from build123d import *

# Parameters (mm, degrees)
BOSS_EXTRUDE1_DEPTH      = 54.6167
BOSS_EXTRUDE1_DEPTH_BACK = 45.3833
SKETCH2_W                = 20
SKETCH2_H                = 20
CUT_EXTRUDE1_DEPTH       = 91
SKETCH3_W                = 20
SKETCH3_H                = 20
CUT_EXTRUDE2_DEPTH       = 91
BOSS_EXTRUDE2_START      = -45.3833
SKETCH1_5_W              = 3
SKETCH1_5_H              = 10
SKETCH1_5_W_2            = 10
SKETCH1_5_H_2            = 3
BOSS_EXTRUDE2_DEPTH      = 80
CUT_EXTRUDE3_REACH       = 92
SKETCH5_R                = 5
SKETCH5_R_2              = 3.4
CUT_EXTRUDE4_REACH       = 92
SKETCH4_R                = 5
SKETCH4_R_2              = 3.4


with BuildPart() as part:
    # Sketch1 → Boss-Extrude1 (new body, two sides)
    with BuildSketch(Plane(origin=(0, 0, 0), x_dir=(1, 0, 0), z_dir=(0, 1, 0))) as boss_extrude1_sk:
        with BuildLine():
            ThreePointArc((45, 25), (39.142135624, 39.142135624), (25, 45))
            Line((25, 45), (-25, 45))
            ThreePointArc((-25, 45), (-39.142135624, 39.142135624), (-45, 25))
            Line((-45, 25), (-45, -25))
            ThreePointArc((-45, -25), (-39.142135624, -39.142135624), (-25, -45))
            Line((-25, -45), (25, -45))
            Line((25, -45), (25, -38))
            Line((25, -38), (15, -38))
            Line((15, -38), (5, -38))
            Line((5, -38), (5, -35))
            Line((5, -35), (-25, -35))
            ThreePointArc((-25, -35), (-32.071067812, -32.071067812), (-35, -25))
            Line((-35, -25), (-35, 25))
            ThreePointArc((-35, 25), (-32.071067812, 32.071067812), (-25, 35))
            Line((-25, 35), (25, 35))
            ThreePointArc((25, 35), (32.071067812, 32.071067812), (35, 25))
            Line((35, 25), (35, -5))
            Line((35, -5), (38, -5))
            Line((38, -5), (38, -15))
            Line((38, -15), (38, -25))
            Line((38, -25), (45, -25))
            Line((45, -25), (45, 25))
        make_face()
    extrude(amount=BOSS_EXTRUDE1_DEPTH)
    extrude(boss_extrude1_sk.sketch, amount=-BOSS_EXTRUDE1_DEPTH_BACK)

    # Sketch2 → Cut-Extrude1 (cut, through all)
    with BuildSketch(Plane(origin=(0, 0, -45), x_dir=(-1, 0, 0), z_dir=(0, 0, -1))):
        with Locations((-35, 44.616700276)):
            Rectangle(SKETCH2_W, SKETCH2_H)
    extrude(amount=-CUT_EXTRUDE1_DEPTH, mode=Mode.SUBTRACT)

    # Sketch3 → Cut-Extrude2 (cut, through all)
    with BuildSketch(Plane.ZY.offset(45)):
        with Locations((35, 44.616700276)):
            Rectangle(SKETCH3_W, SKETCH3_H)
    extrude(amount=-CUT_EXTRUDE2_DEPTH, mode=Mode.SUBTRACT)

    # Sketch1<5> → Boss-Extrude2 (add)
    with BuildSketch(Plane(origin=(0, 0, 0), x_dir=(1, 0, 0), z_dir=(0, 1, 0)).offset(BOSS_EXTRUDE2_START)):
        with BuildLine():
            Line((25, -25), (35, -25))
            Line((35, -25), (35, -15))
            Line((35, -15), (25, -15))
            ThreePointArc((25, -15), (17.928932188, -17.928932188), (15, -25))
            Line((15, -25), (15, -35))
            Line((15, -35), (25, -35))
            Line((25, -35), (25, -25))
        make_face()
        with Locations((36.5, -20)):
            Rectangle(SKETCH1_5_W, SKETCH1_5_H)
        with Locations((20, -36.5)):
            Rectangle(SKETCH1_5_W_2, SKETCH1_5_H_2)
    extrude(amount=BOSS_EXTRUDE2_DEPTH)

    # Sketch5 → Cut-Extrude3 (cut, up to next)
    with BuildSketch(Plane(origin=(0, 0, -45), x_dir=(-1, 0, 0), z_dir=(0, 0, -1)), mode=Mode.PRIVATE) as cut_extrude3_sk1:
        with Locations((0, 9.016700277)):
            Circle(SKETCH5_R)
    cut_extrude3_tool1 = extrude(cut_extrude3_sk1.sketch, amount=-CUT_EXTRUDE3_REACH, mode=Mode.PRIVATE) & part.part
    add(cut_extrude3_tool1.solids().sort_by_distance((0, 9.0167, -45))[0], mode=Mode.SUBTRACT)
    # Sketch5 → Cut-Extrude3 (cut, up to next)
    with BuildSketch(Plane(origin=(0, 0, -45), x_dir=(-1, 0, 0), z_dir=(0, 0, -1)), mode=Mode.PRIVATE) as cut_extrude3_sk2:
        with Locations((0, -25.983299723)):
            Circle(SKETCH5_R)
    cut_extrude3_tool2 = extrude(cut_extrude3_sk2.sketch, amount=-CUT_EXTRUDE3_REACH, mode=Mode.PRIVATE) & part.part
    add(cut_extrude3_tool2.solids().sort_by_distance((0, -25.9833, -45))[0], mode=Mode.SUBTRACT)
    # Sketch5 → Cut-Extrude3 (cut, up to next)
    with BuildSketch(Plane(origin=(0, 0, -45), x_dir=(-1, 0, 0), z_dir=(0, 0, -1)), mode=Mode.PRIVATE) as cut_extrude3_sk3:
        with Locations((16, -25.983299723)):
            Circle(SKETCH5_R_2)
    cut_extrude3_tool3 = extrude(cut_extrude3_sk3.sketch, amount=-CUT_EXTRUDE3_REACH, mode=Mode.PRIVATE) & part.part
    add(cut_extrude3_tool3.solids().sort_by_distance((-16, -25.9833, -45))[0], mode=Mode.SUBTRACT)
    # Sketch5 → Cut-Extrude3 (cut, up to next)
    with BuildSketch(Plane(origin=(0, 0, -45), x_dir=(-1, 0, 0), z_dir=(0, 0, -1)), mode=Mode.PRIVATE) as cut_extrude3_sk4:
        with Locations((-16, -25.983299723)):
            Circle(SKETCH5_R_2)
    cut_extrude3_tool4 = extrude(cut_extrude3_sk4.sketch, amount=-CUT_EXTRUDE3_REACH, mode=Mode.PRIVATE) & part.part
    add(cut_extrude3_tool4.solids().sort_by_distance((16, -25.9833, -45))[0], mode=Mode.SUBTRACT)
    # Sketch5 → Cut-Extrude3 (cut, up to next)
    with BuildSketch(Plane(origin=(0, 0, -45), x_dir=(-1, 0, 0), z_dir=(0, 0, -1)), mode=Mode.PRIVATE) as cut_extrude3_sk5:
        with Locations((-16, 9.016700277)):
            Circle(SKETCH5_R_2)
    cut_extrude3_tool5 = extrude(cut_extrude3_sk5.sketch, amount=-CUT_EXTRUDE3_REACH, mode=Mode.PRIVATE) & part.part
    add(cut_extrude3_tool5.solids().sort_by_distance((16, 9.0167, -45))[0], mode=Mode.SUBTRACT)
    # Sketch5 → Cut-Extrude3 (cut, up to next)
    with BuildSketch(Plane(origin=(0, 0, -45), x_dir=(-1, 0, 0), z_dir=(0, 0, -1)), mode=Mode.PRIVATE) as cut_extrude3_sk6:
        with Locations((16, 9.016700277)):
            Circle(SKETCH5_R_2)
    cut_extrude3_tool6 = extrude(cut_extrude3_sk6.sketch, amount=-CUT_EXTRUDE3_REACH, mode=Mode.PRIVATE) & part.part
    add(cut_extrude3_tool6.solids().sort_by_distance((-16, 9.0167, -45))[0], mode=Mode.SUBTRACT)

    # Sketch4 → Cut-Extrude4 (cut, up to next)
    with BuildSketch(Plane.ZY.offset(45), mode=Mode.PRIVATE) as cut_extrude4_sk1:
        with Locations((0.001556396, 24.616700277)):
            Circle(SKETCH4_R)
    cut_extrude4_tool1 = extrude(cut_extrude4_sk1.sketch, amount=-CUT_EXTRUDE4_REACH, mode=Mode.PRIVATE) & part.part
    add(cut_extrude4_tool1.solids().sort_by_distance((-45, 24.6167, 0.001556))[0], mode=Mode.SUBTRACT)
    # Sketch4 → Cut-Extrude4 (cut, up to next)
    with BuildSketch(Plane.ZY.offset(45), mode=Mode.PRIVATE) as cut_extrude4_sk2:
        with Locations((0.001556396, -10.383299723)):
            Circle(SKETCH4_R)
    cut_extrude4_tool2 = extrude(cut_extrude4_sk2.sketch, amount=-CUT_EXTRUDE4_REACH, mode=Mode.PRIVATE) & part.part
    add(cut_extrude4_tool2.solids().sort_by_distance((-45, -10.3833, 0.001556))[0], mode=Mode.SUBTRACT)
    # Sketch4 → Cut-Extrude4 (cut, up to next)
    with BuildSketch(Plane.ZY.offset(45), mode=Mode.PRIVATE) as cut_extrude4_sk3:
        with Locations((16.001556396, -10.383299723)):
            Circle(SKETCH4_R_2)
    cut_extrude4_tool3 = extrude(cut_extrude4_sk3.sketch, amount=-CUT_EXTRUDE4_REACH, mode=Mode.PRIVATE) & part.part
    add(cut_extrude4_tool3.solids().sort_by_distance((-45, -10.3833, 16.001556))[0], mode=Mode.SUBTRACT)
    # Sketch4 → Cut-Extrude4 (cut, up to next)
    with BuildSketch(Plane.ZY.offset(45), mode=Mode.PRIVATE) as cut_extrude4_sk4:
        with Locations((-15.998443604, -10.383299723)):
            Circle(SKETCH4_R_2)
    cut_extrude4_tool4 = extrude(cut_extrude4_sk4.sketch, amount=-CUT_EXTRUDE4_REACH, mode=Mode.PRIVATE) & part.part
    add(cut_extrude4_tool4.solids().sort_by_distance((-45, -10.3833, -15.998444))[0], mode=Mode.SUBTRACT)
    # Sketch4 → Cut-Extrude4 (cut, up to next)
    with BuildSketch(Plane.ZY.offset(45), mode=Mode.PRIVATE) as cut_extrude4_sk5:
        with Locations((16.001556396, 24.616700277)):
            Circle(SKETCH4_R_2)
    cut_extrude4_tool5 = extrude(cut_extrude4_sk5.sketch, amount=-CUT_EXTRUDE4_REACH, mode=Mode.PRIVATE) & part.part
    add(cut_extrude4_tool5.solids().sort_by_distance((-45, 24.6167, 16.001556))[0], mode=Mode.SUBTRACT)
    # Sketch4 → Cut-Extrude4 (cut, up to next)
    with BuildSketch(Plane.ZY.offset(45), mode=Mode.PRIVATE) as cut_extrude4_sk6:
        with Locations((-15.998443604, 24.616700277)):
            Circle(SKETCH4_R_2)
    cut_extrude4_tool6 = extrude(cut_extrude4_sk6.sketch, amount=-CUT_EXTRUDE4_REACH, mode=Mode.PRIVATE) & part.part
    add(cut_extrude4_tool6.solids().sort_by_distance((-45, 24.6167, -15.998444))[0], mode=Mode.SUBTRACT)


solid = part.part
The listing builds one solid part. Answer for the finished solid, in the listing's coordinates (mm). A direction names the side the tool comes from. Give positions to 0.01 mm unless a question says otherwise; leave off trailing zeros. Order: outer loops, then holes, each group sorted by start corner. A loop starts at its lowest first (then second) coordinate and runs counter-clockwise, first axis right, second up. Notation, with made-up numbers: (17.5, 60.25) - (43.5, 60.25) arc R21 cw to (43.5, 80.25) - close; hole circle Ø3 at (82, 72). An arc over 180 degrees is marked (long way). One line per item, written item: value. Start each with the question number.
1) A cutting plane is placed at C-C on x = -27.5. Give the vertices of the cut face in (y, z).
2) A cutting plane is placed at D-D on x = -16. Give the vertices of the cut face in (y, z), then the cut area to 3 significant figures.
3) Given pin 1 Ø8 at (y, z) = (24.62, 0) entering from -X; pin 2 Ø10.5 at (x, y) = (33, 8.5) entering from -Z; pin 3 Ø10 at (y, z) = (9, -35.5) entering from -X; pin 4 Ø11 at (x, y) = (16, -25.98) entering from -Z, each flat-ended and moving along its own axis, determine where each tip first touches the part or whether it passes through.
4) The mould has two halves that part along X. Classify faces 1 (the face through (-35, 5, 0)), 2 (the face through (-39.297, -4.823, 38.986)), 3 (the face through (18.51, 11.31, -40.07)), 4 (the face through (0, -5, 45)): released by +X, released by -X, zero draft, split by the parting line, or undercut.
5) A cutting plane is placed at B-B on x = 0. Give the vertices of the cut face in (y, z).
6) A tool of negligible diameter and unlimited length cuts with its end or side. For faces 5 (the face through (36, -5, 5)), 6 (the face through (25, 44, -40)), 7 (the face through (-40, 44, 25)), 8 (the face through (-40.07, 23.31, -12.86)), 9 (the face through (0.651, 13.974, -40.07)), from which of +Z, -Z, +X, -X, +Y, -Y can it reach the whole face along a straight path? Write none if from no direction.
7) Find the intervals of material crossed by L1, parallel to Y at x = 0, z = -41; L2, parallel to Y at x = -16, z = -41; L3, parallel to X at y = -19.5, z = 11.5, in increasing order.
8) A cutting plane is placed at A-A on z = -21. Give the vertices of the cut face in (x, y).
Answer sheet:
1. outline: (-45.38, -44.84) - (54.62, -44.84) - (54.62, -34.68) - (-45.38, -34.68) - close; (-45.38, 34.68) - (34.62, 34.68) - (34.62, 44.84) - (-45.38, 44.84) - close
2. outline: (-45.38, -45) - (-29.38, -45) - (-29.38, -35) - (-45.38, -35) - close; (-45.38, 35) - (34.62, 35) - (34.62, 45) - (-45.38, 45) - close; (-22.58, -45) - (5.62, -45) - (5.62, -35) - (-22.58, -35) - close; (12.42, -45) - (54.62, -45) - (54.62, -35) - (12.42, -35) - close
2. area: 1,660 mm2
3. pin 1: stops at x = 35
3. pin 2: stops at z = -44.81
3. pin 3: stops at x = -44.23
3. pin 4: stops at z = -45
4. face 1: undercut
4. face 2: released by -X
4. face 3: undercut
4. face 4: zero draft
5. outline: (-45.38, -45) - (-30.98, -45) - (-30.98, -35) - (-45.38, -35) - close; (-45.38, 35) - (34.62, 35) - (34.62, 45) - (-45.38, 45) - close; (-20.98, -45) - (4.02, -45) - (4.02, -35) - (-20.98, -35) - close; (14.02, -45) - (54.62, -45) - (54.62, -35) - (14.02, -35) - close
6. face 5: +Y, -Y
6. face 6: +Z, -Z, +X, +Y
6. face 7: +Z, +X, -X, +Y
6. face 8: -X
6. face 9: -Z
7. L1: y = -45.38 to -30.98, -20.98 to 4.02, 14.02 to 54.62
7. L2: y = -45.38 to -29.38, -22.58 to 5.62, 12.42 to 54.62
7. L3: x = -45 to -35, 38 to 45
8. outline: (-45, -45.38) - (-35, -45.38) - (-35, 54.62) - (-45, 54.62) - close; (35, -45.38) - (45, -45.38) - (45, 34.62) - (35, 34.62) - close
